Verification items for the finished model (mm, model axes). A direction names the side the tool comes from. Give positions to 0.01 mm unless a question says otherwise; leave off trailing zeros. Loops run counter-clockwise (first coordinate to the right, second up) from the corner with the lowest first, then second, coordinate; pieces in that order, holes last. Notation, with made-up numbers: (89.5, -8) - (94.5, -8) arc R11 ccw to (94.5, 5) - close; hole circle Ø10 at (52, -14). An arc over 180 degrees is marked (long way). One line per question, with ' | ' between items. Start each with the question number.
1. Mould release check, pull along Y, two halves, no side actions. Record for faces 1 (the face through (-3.47, -15.62, 3.36)), 2 (the face through (-6, 12, 0)), 3 (the face through (-14.985, 0.66, 3.958)): +Y half, -Y half, draft (parallel to the pull), parting line (faces both ways), or undercut.
2. Depth check by flat-ended pin: pin 1 Ø9 at (x, y) = (-5.5, 2.5) entering from +Z; pin 2 Ø2 at (x, z) = (8, 6) entering from +Y; pin 3 Ø8 at (x, y) = (1.5, 8.5) entering from -Z. Enter the tip coordinate at first touch or a pass-through.
3. Section check A-A, the plane x = 0. Enter the section's corners in (y, z), then the cut area to 3 significant figures.
4. Section check C-C, the plane z = 4.25. Enter the section's corners in (x, y), then the cut area to 3 significant figures.
5. Thickness scan on line 1 along Y through (x, z) = (0, 5.35); line 2 along Z through (x, y) = (-2.5, 11.5); line 3 along X through (y, z) = (5, 6). Record the ranges inside material, lowest first. Write a range as from..to.
6. Tool access check on faces 4 (the face through (0, 0, 1)), 5 (the face through (-8, 13, 7)), 6 (the face through (0, 0, 0.1)). Record the directions out of +Z, -Z, +X, -X, +Y, -Y that give a thin tool (end or side, any length) a straight path to the whole face; none if there is none.
from build123d import *

# Parameters (mm, degrees)
SKICA1_R                 = 16
P_IDAT_VYSUNUT_M1_DEPTH  = 7
SKO_EPINA1_T             = -1
SKICA2_R                 = 13
ODEBRAT_VYSUNUT_M1_DEPTH = 0.1
ZKOSEN_1_SIZE            = 0.5
ZKOSEN_2_SIZE            = 0.3


with BuildPart() as part:
    # Skica1 → Přidat vysunutím1 (new body)
    with BuildSketch(Plane.XY):
        Circle(SKICA1_R)
    extrude(amount=P_IDAT_VYSUNUT_M1_DEPTH)

    # Skořepina1
    sko_epina1_openings = [part.faces().sort_by_distance(p)[0] for p in [
        (0, 0, 7),
    ]]
    offset(amount=SKO_EPINA1_T, openings=sko_epina1_openings, kind=Kind.INTERSECTION)

    # Skica2 → Odebrat vysunutím1 (cut)
    with BuildSketch(Plane(origin=(0, 0, 0), x_dir=(-1, 0, 0), z_dir=(0, 0, -1))):
        Circle(SKICA2_R)
    extrude(amount=-ODEBRAT_VYSUNUT_M1_DEPTH, mode=Mode.SUBTRACT)

    # Zkosení1
    zkosen_1_edges = [part.edges().sort_by_distance(p)[0] for p in [
        (-16, 0, 7),
    ]]
    chamfer(zkosen_1_edges, length=ZKOSEN_1_SIZE)

    # Zkosení2
    zkosen_2_edges = [part.edges().sort_by_distance(p)[0] for p in [
        (-16, 0, 0),
    ]]
    chamfer(zkosen_2_edges, length=ZKOSEN_2_SIZE)


solid = part.part
Results list:
1) face 1: parting line | face 2: draft | face 3: undercut
2) pin 1: z = 1 | pin 2: y = 14.39 | pin 3: z = 0.1
3) outline: (-16, 0.3) - (-15.7, 0) - (-13, 0) - (-13, 0.1) - (13, 0.1) - (13, 0) - (15.7, 0) - (16, 0.3) - (16, 6.5) - (15.5, 7) - (15, 7) - (15, 1) - (-15, 1) - (-15, 7) - (-15.5, 7) - (-16, 6.5) - close | area: 41.1 mm²
4) outline: circle Ø32 at (0, 0); hole circle Ø30 at (0, 0) | area: 97.4 mm²
5) line 1: -16..-15, 15..16 | line 2: 0.1..1 | line 3: -15.2..-14.14, 14.14..15.2
6) face 4: +Z | face 5: +Z, +X, -X, +Y, -Y | face 6: -Z
